Check sheet for the modelled part. Datum: model origin and axes. Units: mm. Face numbers are marked on the shaded views. Give positions to 0.01 mm unless a question says otherwise; leave off trailing zeros. Order: outer loops, then holes, each group sorted by start corner. A loop starts at its lowest first (then second) coordinate and runs counter-clockwise, first axis right, second up.
Item 1: Material ranges on line 1 along Y through (x, z) = (-135, -4.75); line 2 along X through (y, z) = (11.5, -19); line 3 along X through (y, z) = (1.5, -7), recorded low to high.
Item 2: Sectioned sample at D-D on y = 23.75. Record the boundary of the cut face in (x, z), and give its area (3 significant figures).
Item 3: Gauge pin test, flat ends, axial feed: P1, Ø1, axis at y = 8, z = -13.5, coming from the +X side; P2, Ø1, axis at y = 13.5, z = -9.5, coming from the +X side; P3, Ø4, axis at y = 22, z = -9, coming from the -X side. Record the tip position at first contact, or that the pin passes through.
Item 4: Sectioned sample at B-B on z = -12.75. Record the boundary of the cut face in (x, y), and give its area (3 significant figures).
Item 5: Sectioned sample at A-A on x = -128. Record the boundary of the cut face in (y, z).
Item 6: Sectioned sample at C-C on z = -18.25. Record the boundary of the cut face in (x, y).
Item 7: Release check for a two-part mould opening along Z. For the marked faces 1, 2, 3 and 4 record: released by +Z, released by -Z, zero draft, split by the parting line, or undercut.
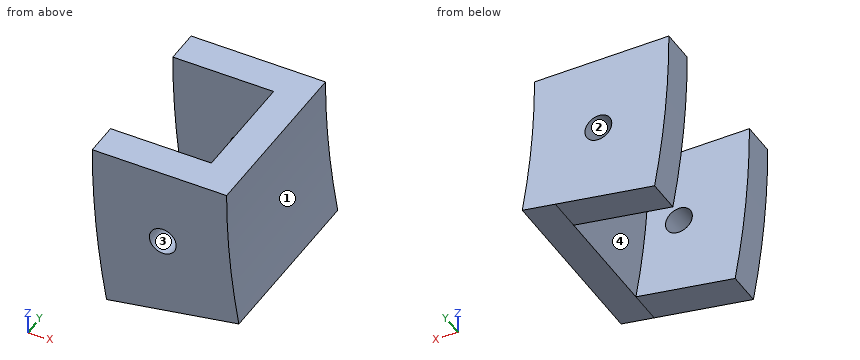
Autodesk Inventor part; units mm, degrees
ref_plane "YZ Plane" through (0, 0, 0) normal (1, 0, 0) x (0, 1, 0)
ref_plane "XZ Plane" through (0, 0, 0) normal (0, 1, 0) x (-1, 0, 0)
ref_plane "XY Plane" through (0, 0, 0) normal (0, 0, 1) x (1, 0, 0)
sketch "Sketch1" plane through (0, 0, 0) normal (0, 1, 0) x (-1, 0, 0)
  line L0 (0, 0) -> (125, 0) construction
  line L1 (0, 0) -> (125, 0) construction
  line L2 (0, 0) -> (123.101, -21.706) construction
  line L3 (0, 0) -> (300, 0) construction
  line L4 (0, 0) -> (300, 0) construction
  line L5 (140, 0) -> (125, 0)
  line L6 (137.8731, -24.3107) -> (123.101, -21.706)
  line L7 (124.5243, -10.8945) -> (129.5053, -11.3302)
  circle A0 centre (129.5053, -11.3302) radius 2
  arc A1 (137.8731, -24.3107) -> (140, 0) centre (0, 0) ccw
  arc A2 (123.101, -21.706) -> (124.5243, -10.8945) centre (0, 0) ccw
  arc A3 (124.5243, -10.8945) -> (125, 0) centre (0, 0) ccw
  dimension "d1" = 0
  dimension "d2" = 10
  dimension "d4" = 0
  dimension "d7" = 5
  dimension "d8" = 5
  dimension "d9" = 4
  dimension "d28" = 140
  dimension "d29" = 125
  dimension "d31" = 14.7721
extrude "Extrusion1" add sketch "Sketch1" along normal blind 5
sketch "Sketch3" plane through (0, 5, 0) normal (0, 1, 0) x (1, 0, 0)
  arc A0 (-123.101, 21.706) -> (-125, 0) centre (0, 0) ccw
  arc A1 (-123.101, 21.706) -> (-125, 0) centre (0, 0) ccw
  arc A2 (-118.1769, 20.8378) -> (-120, 0) centre (0, 0) ccw
  line L0 (0, 0) -> (-118.1769, 20.8378) construction
  line L1 (0, 0) -> (-120, 0) construction
  line L2 (-123.101, 21.706) -> (-118.1769, 20.8378)
  line L3 (-125, 0) -> (-120, 0)
  dimension "d33" = 120
  dimension "d34" = 10
extrude "Extrusion4" add sketch "Sketch3" along normal blind 27 from surface at -5
pattern_linear "Rectangular Pattern3" count 2 spacing 22 along (0, 1, 0) of "Extrusion1"
properties part number "Inner_mount"
Report:
1. line 1: y = 0 to 5, 22 to 27
1. line 2: x = -123.55 to -118.49
1. line 3: x = -139.82 to -119.8
2. outline: (-140, 0) arc R140 ccw to (-137.87, -24.31) - (-123.1, -21.71) - (-118.18, -20.84) arc R120 cw to (-120, 0) - close; hole circle Ø4 at (-129.51, -11.33)
2. area: 441 mm2
3. P1: stops at x = -119.18
3. P2: stops at x = -119.58
3. P3: stops at x = -139.82
4. outline: (-139.42, 0) - (-130.91, 0) - (-130.91, 5) - (-139.42, 5) - close; (-139.42, 22) - (-130.91, 22) - (-130.91, 27) - (-139.42, 27) - close; (-128.1, 0) - (-119.32, 0) - (-119.32, 27) - (-128.1, 27) - (-128.1, 22) - (-124.35, 22) - (-124.35, 5) - (-128.1, 5) - close
4. area: 258 mm2
5. outline: (0, -22.57) - (5, -22.57) - (5, -12.65) - (0, -12.65) - close; (0, -10.01) - (5, -10.01) - (5, 0) - (0, 0) - close; (22, -22.57) - (27, -22.57) - (27, -12.65) - (22, -12.65) - close; (22, -10.01) - (27, -10.01) - (27, 0) - (22, 0) - close
6. outline: (-138.81, 0) - (-118.6, 0) - (-118.6, 27) - (-138.81, 27) - (-138.81, 22) - (-123.66, 22) - (-123.66, 5) - (-138.81, 5) - close
7. face 1: released by +Z
7. face 2: undercut
7. face 3: undercut
7. face 4: released by -Z
